Could you check a few things on this model? Use its own coordinates, in mm. Face numbers are marked on the shaded views. A direction names the side the tool comes from. Round coordinates to 2 decimals unless told otherwise and drop trailing zeros. Order: outer loops, then holes, each group sorted by start corner. A loop starts at its lowest first (then second) coordinate and runs counter-clockwise, first axis right, second up. Notation, with made-up numbers: M 88.25,7 L 114.25,7 A13 cw 114.25,32 Z; hole C 51.5,64.5 d9. An arc over 180 degrees is marked long. Write each question's results on one line, items separated by ' | '. Start each with the question number.
1. Suppose I cut it at A-A on z = -18.5. Write out the boundary of the cut face in (x, y).
2. Suppose I cut it at C-C on x = 3. Write out the boundary of the cut face in (y, z).
3. Suppose I cut it at D-D on z = -4.5. Write out the boundary of the cut face in (x, y).
4. I'm going to push flat-ended pins straight in: pin 1 (8 mm diameter, centred on x = 42, y = -9, fed in from -Z); pin 2 (3 mm diameter, centred on y = -8, z = -58, fed in from +X); pin 3 (1.5 mm diameter, centred on y = -7, z = -47, fed in from +X); pin 4 (12 mm diameter, centred on x = 9, z = -31, fed in from -Y). Where does each tip first touch, or does it pass through?
5. Please list where these lines run through material, in increasing order: L1, parallel to Z at x = 15.5, y = -7.25; L2, parallel to Z at x = 1, y = -4; L3, parallel to Z at x = 25, y = -2.5.
6. We'd pull the mould along X, two halves only. Please class the marked faces 6, 7 and 8: released by +X, released by -X, zero draft, split by the parting line, or undercut.
7. For the marked faces 1, 2, 3, 4 and 5, which set-ups out of +Z, -Z, +X, -X, +Y, -Y let a thin tool reach every point of the face, with its end or its side?
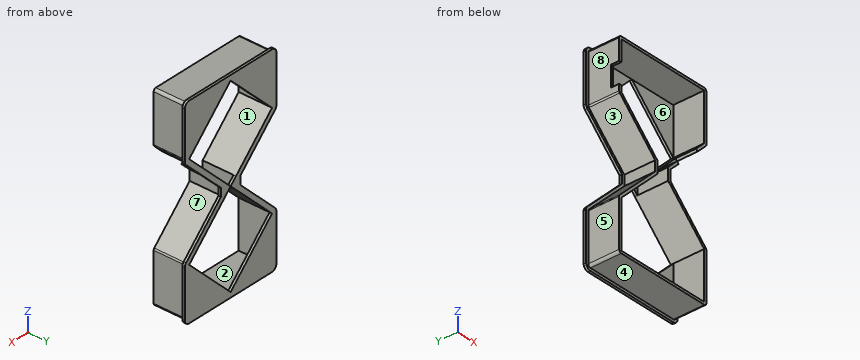
from build123d import *

# Parameters (mm, degrees)
EXTRUDE_2_DEPTH      = 1.2
EXTRUDE_4_DEPTH      = 15
CUT_EXTRUDE_13_REACH = 109.14
CUT_EXTRUDE_15_REACH = 109.14
CUT_EXTRUDE_16_REACH = 109.14
CUT_EXTRUDE_17_REACH = 73.673


with BuildPart() as part:
    # 草图1 → 凸台-拉伸2 (new body)
    with BuildSketch(Plane(origin=(0, 0, 0), x_dir=(1, 0, 0), z_dir=(0, 1, 0))):
        with BuildLine():
            Line((-2.399264051, 68.999900529), (-2.399264051, 91.999900529))
            ThreePointArc((-2.399264051, 91.999900529), (-1.696320326, 93.696956804), (0.000735949, 94.399900529))
            Line((0.000735949, 94.399900529), (46.000735949, 94.399900529))
            ThreePointArc((46.000735949, 94.399900529), (47.697792224, 93.696956804), (48.400735949, 91.999900529))
            Line((48.400735949, 91.999900529), (48.400735949, 68.999900529))
            ThreePointArc((48.400735949, 68.999900529), (48.218046827, 68.081460292), (47.697792224, 67.302844254))
            Line((47.697792224, 67.302844254), (28.40092775, 48.00597978))
            Line((28.40092775, 48.00597978), (28.40092775, 43.99420488))
            Line((28.40092775, 43.99420488), (47.697792224, 24.697340406))
            ThreePointArc((47.697792224, 24.697340406), (48.218046827, 23.918724369), (48.400735949, 23.000284131))
            Line((48.400735949, 23.000284131), (48.400735949, 0.000284131))
            ThreePointArc((48.400735949, 0.000284131), (47.681245751, -1.713158837), (45.954163612, -2.399263955))
            Line((45.954163612, -2.399263955), (0.000735672, -2.399263955))
            ThreePointArc((0.000735672, -2.399263955), (-1.696376241, -1.696695528), (-2.399264051, 0.000284131))
            Line((-2.399264051, 0.000284131), (-2.399264051, 23.000284131))
            ThreePointArc((-2.399264051, 23.000284131), (-2.216574929, 23.918724369), (-1.696320326, 24.697340406))
            Line((-1.696320326, 24.697340406), (17.600544148, 43.99420488))
            Line((17.600544148, 43.99420488), (17.600544148, 48.00597978))
            Line((17.600544148, 48.00597978), (-1.696320326, 67.302844254))
            ThreePointArc((-1.696320326, 67.302844254), (-2.216574929, 68.081460292), (-2.399264051, 68.999900529))
        make_face()
    extrude(amount=EXTRUDE_2_DEPTH)

    # 草图3 → 凸台-拉伸4 (add)
    with BuildSketch(Plane.XZ):
        with BuildLine():
            Line((0, -93.138725211), (46, -93.138725211))
            ThreePointArc((46, -93.138725211), (46.848528137, -92.787253348), (47.2, -91.938725211))
            Line((47.2, -91.938725211), (47.2, -68.938725211))
            ThreePointArc((47.2, -68.938725211), (47.108655439, -68.479505092), (46.848528137, -68.090197073))
            Line((46.848528137, -68.090197073), (27.200191801, -48.441860737))
            Line((27.200191801, -48.441860737), (27.200191801, -43.496864474))
            Line((27.200191801, -43.496864474), (46.848528137, -23.848528137))
            ThreePointArc((46.848528137, -23.848528137), (47.108655439, -23.459220119), (47.2, -23))
            Line((47.2, -23), (47.2, 0))
            ThreePointArc((47.2, 0), (46.848528137, 0.848528137), (46, 1.2))
            Line((46, 1.2), (0, 1.2))
            ThreePointArc((0, 1.2), (-0.848528137, 0.848528137), (-1.2, 0))
            Line((-1.2, 0), (-1.2, -23))
            ThreePointArc((-1.2, -23), (-1.108655439, -23.459220119), (-0.848528137, -23.848528137))
            Line((-0.848528137, -23.848528137), (18.799808199, -43.496864474))
            Line((18.799808199, -43.496864474), (18.799808199, -48.441860737))
            Line((18.799808199, -48.441860737), (-0.848528137, -68.090197073))
            ThreePointArc((-0.848528137, -68.090197073), (-1.108655439, -68.479505092), (-1.2, -68.938725211))
            Line((-1.2, -68.938725211), (-1.2, -91.938725211))
            ThreePointArc((-1.2, -91.938725211), (-0.848528137, -92.787253348), (0, -93.138725211))
        make_face()
        Polygon((0, -23), (19.999808199, -42.999808199), (19.999808199, -48.938917012), (0, -68.938725211), (0, -91.938725211), (46, -91.938725211), (46, -68.938725211), (26.000191801, -48.999808199), (26.000191801, -42.999808199), (46, -23), (46, 0), (0, 0), align=None, mode=Mode.SUBTRACT)
    extrude(amount=EXTRUDE_4_DEPTH)

    # 草图11 → 切除-拉伸13 (cut, up to next)
    with BuildSketch(Plane(origin=(0, 0, 0), x_dir=(-1, 0, 0), z_dir=(0, -1, 0)), mode=Mode.PRIVATE) as cut_extrude_13_sk1:
        Polygon((-19.999808199, 42.999808199), (-23, 45.969362605), (-26.000191801, 42.999808199), (-46, 23), (-23, 0), (0, 23), align=None)
    cut_extrude_13_tool1 = extrude(cut_extrude_13_sk1.sketch, amount=-CUT_EXTRUDE_13_REACH, mode=Mode.PRIVATE) & part.part
    add(cut_extrude_13_tool1.solids().sort_by_distance((23, 0, -22.998089))[0], mode=Mode.SUBTRACT)

    # 草图16 → 切除-拉伸15 (cut, up to next)
    with BuildSketch(Plane.XZ, mode=Mode.PRIVATE) as cut_extrude_15_sk1:
        Polygon((0, -68.938725211), (23, -91.938725211), (46, -68.938725211), (26.000191801, -48.999808199), (23.071072637, -46.041151936), (23.071072637, -45.899015749), (22.928927363, -45.899015749), (22.928927363, -46.039709462), (19.999808199, -48.938917012), align=None)
    cut_extrude_15_tool1 = extrude(cut_extrude_15_sk1.sketch, amount=-CUT_EXTRUDE_15_REACH, mode=Mode.PRIVATE) & part.part
    add(cut_extrude_15_tool1.solids().sort_by_distance((22.99426, 0, -68.949789))[0], mode=Mode.SUBTRACT)

    # 草图17 → 切除-拉伸16 (cut, up to next)
    with BuildSketch(Plane(origin=(0, 0, 0), x_dir=(0, 0, -1), z_dir=(1, 0, 0)), mode=Mode.PRIVATE) as cut_extrude_16_sk1:
        Polygon((10, -11), (10, -15), (15, -15), (20, -15), (20, -11), (15, -11), align=None)
    cut_extrude_16_tool1 = extrude(cut_extrude_16_sk1.sketch, amount=-CUT_EXTRUDE_16_REACH, mode=Mode.PRIVATE) & part.part
    add(cut_extrude_16_tool1.solids().sort_by_distance((0, -13, -15))[0], mode=Mode.SUBTRACT)

    # 草图18 → 切除-拉伸17 (cut, up to next)
    with BuildSketch(Plane(origin=(35.348528137, 0, -35.348528137), x_dir=(-0.707106781186532, 0, -0.707106781186563), z_dir=(0.707106781186563, 0, -0.707106781186532)), mode=Mode.PRIVATE) as cut_extrude_17_sk1:
        Polygon((-2.369984105, -15), (5.130015895, -15), (5.130015895, -5), (-9.869984105, -5), (-9.869984105, -15), align=None)
    cut_extrude_17_tool1 = extrude(cut_extrude_17_sk1.sketch, amount=-CUT_EXTRUDE_17_REACH, mode=Mode.PRIVATE) & part.part
    add(cut_extrude_17_tool1.solids().sort_by_distance((37.02436, -10, -33.672696))[0], mode=Mode.SUBTRACT)


solid = part.part
Filled sheet:
1) outline: M -2.4,0 L -1.2,0 L -1.2,-11 L 0,-11 L 0,0 L 4.5,0 L 4.5,1.2 L -2.4,1.2 Z; M 41.5,0 L 46,0 L 46,-15 L 47.2,-15 L 47.2,0 L 48.4,0 L 48.4,1.2 L 41.5,1.2 Z
2) outline: M -15,-93.14 L 0,-93.14 L 0,-94.4 L 1.2,-94.4 L 1.2,-71.94 L 0,-71.94 L 0,-91.94 L -15,-91.94 Z; M -15,-65.94 L 1.2,-65.94 L 1.2,-62.61 L 0,-62.61 L 0,-64.24 L -15,-64.24 Z; M -15,-27.7 L 0,-27.7 L 0,-29.39 L 1.2,-29.39 L 1.2,-26 L -15,-26 Z; M -15,0 L 0,0 L 0,-20 L 1.2,-20 L 1.2,2.4 L 0,2.4 L 0,1.2 L -15,1.2 Z
3) outline: M -2.4,0 L -1.2,0 L -1.2,-15 L 0,-15 L 0,0 L 18.5,0 L 18.5,1.2 L -2.4,1.2 Z; M 27.5,0 L 46,0 L 46,-15 L 47.2,-15 L 47.2,0 L 48.4,0 L 48.4,1.2 L 27.5,1.2 Z
4) pin 1: stops at z = -93.14 | pin 2: stops at x = 38.26 | pin 3: stops at x = 27.2 | pin 4: stops at y = -15
5) L1: z = -93.14 to -91.94, -53.44 to -51.74, -40.2 to -38.5, 0 to 1.2 | L2: z = -93.14 to -91.94, -67.94 to -66.24, -25.7 to -24, 0 to 1.2 | L3: z = -93.14 to -91.94, 0 to 1.2
6) face 6: undercut | face 7: released by +X | face 8: released by -X
7) face 1: +Y, -Y | face 2: -Y | face 3: -X, -Y | face 4: -Z, +X, -X, -Y | face 5: +Z, -Z, -X, -Y
